Verification items for the finished model (mm, model axes). Face numbers are marked on the shaded views. A direction names the side the tool comes from. Give positions to 0.01 mm unless a question says otherwise; leave off trailing zeros. Answer in a Markdown table with one row per item.
```python
from build123d import *

# Parameters (mm, degrees)
F0_R         = 11.25
F1_DEPTH     = 2.175
F2_R         = 11.25
F3_DEPTH     = 1.5
F5_W         = 11
F5_H         = 5.5
F6_DEPTH     = 21
F7_W         = 11
F7_H         = 5.5
F8_DEPTH     = 21
F9_W         = 11
F9_H         = 5
F10_DEPTH    = 21
F11_T1_DEPTH = 15.005727874
F12_R        = 1
F13_R        = 0.5
F14_R        = 0.5
F15_R        = 0.5
F16_R        = 0.5
F17_R        = 0.5
F18_R        = 0.5
F19_R        = 0.5
F20_R        = 1


# Not quite as in the source:
# - a fillet or chamfer that OpenCascade refuses, or shapes differently, is made with other operations: its cross-section is extruded or revolved along the edge and cut away or added


with BuildPart() as f1:
    # F0 (on Top) → F1 (new body, symmetric)
    with BuildSketch(Plane.XY):
        Polygon((-2.2081266769, 22.9882037122), (-21.0124317406, 9.5818080591), (-18.8043050636, -13.4063956531), (2.2081266769, -22.9882037122), (21.0124317406, -9.5818080591), (18.8043050636, 13.4063956531), align=None)
        Circle(F0_R, mode=Mode.SUBTRACT)
        Polygon((-28.2205584175, 29.0052973062), (-21.0124317406, 9.5818080591), (-2.2081266769, 22.9882037122), (-18.2205584175, 36.1347262363), align=None)
        Polygon((2.2081266769, -22.9882037122), (-18.8043050636, -13.4063956531), (-22.1833116707, -33.8468295789), (-11.0090451027, -38.9423691517), align=None)
        Polygon((39.2296035202, 9.9370718455), (18.8043050636, 13.4063956531), (21.0124317406, -9.5818080591), (40.4038700882, -2.2878966574), align=None)
    extrude(amount=F1_DEPTH, both=True)

    # F2 (on face) → F3 (join)
    with BuildSketch(Plane.XY.offset(2.175)):
        Polygon((-18.8043050636, -13.4063956531), (-22.1833116707, -33.8468295789), (-11.0090451027, -38.9423691517), (2.2081266769, -22.9882037122), (21.0124317406, -9.5818080591), (40.4038700882, -2.2878966574), (39.2296035202, 9.9370718455), (18.8043050636, 13.4063956531), (-2.2081266769, 22.9882037122), (-18.2205584175, 36.1347262363), (-28.2205584175, 29.0052973062), (-21.0124317406, 9.5818080591), align=None)
        Circle(F2_R, mode=Mode.SUBTRACT)
    extrude(amount=F3_DEPTH)

    # F4: F1 across plane


with BuildPart() as f1_1:
    add(f1.part)
    add(f1.part.mirror(Plane.XY))

    # F5 (on face) → F6 (cut)
    with BuildSketch(Plane(origin=(39.8167368042, 3.824587594, 0), x_dir=(-0.0956146899, 0.9954184201, 0), z_dir=(0.9954184201, 0.0956146899, 0))):
        with Locations((0.0001179833, 0.075)):
            Rectangle(F5_W, F5_H)
    extrude(amount=-F6_DEPTH, mode=Mode.SUBTRACT)

    # F7 (on face) → F8 (cut)
    with BuildSketch(Plane(origin=(-23.2205584175, 32.5700117712, 0), x_dir=(-0.8142502943, -0.5805139604, 0), z_dir=(-0.5805139604, 0.8142502943, 0))):
        with Locations((0.0003820167, 0)):
            Rectangle(F7_W, F7_H)
    extrude(amount=-F8_DEPTH, mode=Mode.SUBTRACT)

    # F9 (on face) → F10 (cut)
    with BuildSketch(Plane(origin=(-16.5961783867, -36.3945993653, 0), x_dir=(0.9098649841, -0.4149044597, 0), z_dir=(-0.4149044597, -0.9098649841, 0))):
        with Locations((0.0001179833, 0)):
            Rectangle(F9_W, F9_H)
    extrude(amount=-F10_DEPTH, mode=Mode.SUBTRACT)

    # F11: fillet of radius 2 on 6 edges, made by hand

    # F11_s2 → F11_t1 (cut)
    with BuildSketch(Plane.XY.offset(-7.502863937)):
        with BuildLine():
            ThreePointArc((-17.0371647686, 35.1631366918), (-18.2382120361, 35.6162160874), (-19.4672941524, 35.2458748546))
            Line((-19.4672941524, 35.2458748546), (-18.2205584175, 36.1347262363))
            Line((-18.2205584175, 36.1347262363), (-17.0371647686, 35.1631366918))
        make_face()
        with BuildLine():
            ThreePointArc((-27.6878441198, 27.5698105427), (-27.7246206597, 28.8529484789), (-26.9738226827, 29.8941486878))
            Line((-26.9738226827, 29.8941486878), (-28.2205584175, 29.0052973062))
            Line((-28.2205584175, 29.0052973062), (-27.6878441198, 27.5698105427))
        make_face()
        with BuildLine():
            ThreePointArc((-21.9335872676, -32.336185844), (-21.7254419003, -33.6028629865), (-20.7901759265, -34.4821087062))
            Line((-20.7901759265, -34.4821087062), (-22.1833116707, -33.8468295789))
            Line((-22.1833116707, -33.8468295789), (-21.9335872676, -32.336185844))
        make_face()
        with BuildLine():
            ThreePointArc((-12.4021808468, -38.3070900243), (-11.125076027, -38.4367000411), (-10.0322342476, -37.7632816551))
            Line((-10.0322342476, -37.7632816551), (-11.0090451027, -38.9423691517))
            Line((-11.0090451027, -38.9423691517), (-12.4021808468, -38.3070900243))
        make_face()
        with BuildLine():
            ThreePointArc((38.9707520362, -2.8269508478), (39.9636539364, -2.0133531008), (40.2574700789, -0.7637661484))
            Line((40.2574700789, -0.7637661484), (40.4038700882, -2.2878966574))
            Line((40.4038700882, -2.2878966574), (38.9707520362, -2.8269508478))
        make_face()
        with BuildLine():
            ThreePointArc((37.7200783674, 10.1934711124), (38.8496966867, 9.5837515621), (39.3760035295, 8.4129413364))
            Line((39.3760035295, 8.4129413364), (39.2296035202, 9.9370718455))
            Line((39.2296035202, 9.9370718455), (37.7200783674, 10.1934711124))
        make_face()
    extrude(amount=F11_T1_DEPTH, mode=Mode.SUBTRACT)

    # F12
    f12_edges = [f1_1.edges().sort_by_distance(p)[0] for p in [
        (-16.596178, -36.394599, 3.675),
    ]]
    fillet(f12_edges, radius=F12_R)

    # F13
    f13_edges = [f1_1.edges().sort_by_distance(p)[0] for p in [
        (29.991592, -6.204379, 3.675),
    ]]
    fillet(f13_edges, radius=F13_R)

    # F14
    f14_edges = [f1_1.edges().sort_by_distance(p)[0] for p in [
        (-23.220558, 32.570012, 3.675),
    ]]
    fillet(f14_edges, radius=F14_R)

    # F15
    f15_edges = [f1_1.edges().sort_by_distance(p)[0] for p in [
        (-19.908368, -1.912294, 3.675),
        (11.610279, -16.285006, 3.675),
        (8.298089, 18.1973, 3.675),
    ]]
    fillet(f15_edges, radius=F15_R)

    # F16
    f16_edges = [f1_1.edges().sort_by_distance(p)[0] for p in [
        (-24.350138, 18.575809, -3.675),
    ]]
    fillet(f16_edges, radius=F16_R)

    # F17
    f17_edges = [f1_1.edges().sort_by_distance(p)[0] for p in [
        (28.262192, 11.799933, -3.675),
    ]]
    fillet(f17_edges, radius=F17_R)

    # F18
    f18_edges = [f1_1.edges().sort_by_distance(p)[0] for p in [
        (-3.912054, -30.375743, -3.675),
    ]]
    fillet(f18_edges, radius=F18_R)

    # F19
    f19_edges = [f1_1.edges().sort_by_distance(p)[0] for p in [
        (-19.908368, -1.912294, -3.675),
        (11.610279, -16.285006, -3.675),
        (8.298089, 18.1973, -3.675),
    ]]
    fillet(f19_edges, radius=F19_R)

    # F20
    f20_edges = [f1_1.edges().sort_by_distance(p)[0] for p in [
        (-11.25, 0, 3.675),
        (-11.25, 0, -3.675),
    ]]
    fillet(f20_edges, radius=F20_R)


solid = f1_1.part
```
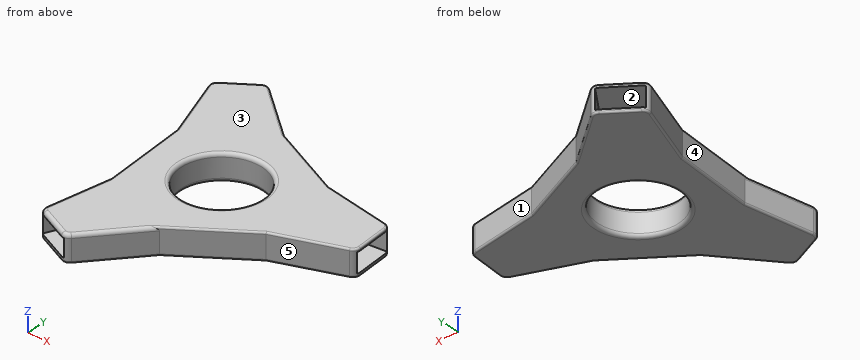
Item 1: Go/stop test with flat-tipped pins: pin 1 (1 mm diameter, centred on y = 9, z = -0.5, fed in from +X); pin 2 (2 mm diameter, centred on x = -9.5, z = -1, fed in from -Y). Record where each tip stops, or that it passes through.
Reported:
| item | result |
|---|---|
| pin 1 | stops at x = 39.08 |
| pin 2 | stops at y = -38.18 |
Item 2: Tool access check on the marked faces 4 and 5. Record the directions out of +Z, -Z, +X, -X, +Y, -Y that give a thin tool (end or side, any length) a straight path to the whole face; none if there is none.
Reported:
| item | result |
|---|---|
| face 4 | +Z, -Z, -X |
| face 5 | +Z, -Z, +X, -Y |
Item 3: Sectioned sample at B-B (x = -8). State how many separate pieces and enclosed holes the cut face has, and give its area (3 significant figures).
Reported:
| item | result |
|---|---|
| separate pieces | 2 |
| enclosed holes | 2 |
| area | 261 mm^2 |
Item 4: Release check for a two-part mould opening along Z. For the marked faces 1, 2 and 3 record: released by +Z, released by -Z, zero draft, split by the parting line, or undercut.
Reported:
| item | result |
|---|---|
| face 1 | zero draft |
| face 2 | undercut |
| face 3 | released by +Z |
Item 5: Scan lines: L1, parallel to Z at x = -16, y = -26 (3 decimals); L2, parallel to X at y = 15, z = -1.5; L3, parallel to X at y = -25, z = 1.5. Record each from-to range of solid material in increasing order. Write a range as [from, to].
Reported:
| item | result |
|---|---|
| L1 | z = [-3.675, -2.5], [2.5, 3.675] |
| L2 | x = [-23.02, -17.45], [-11.69, 15.31] |
| L3 | x = [-20.72, -17.44], [-5.36, 0.54] |
